```python
from build123d import *

# Parameters (mm, degrees)
SKETCH1_W                                    = 122
SKETCH1_H                                    = 43
BOSS_EXTRUDE1_DEPTH                          = 1.8
SKETCH2_W                                    = 9.05
SKETCH2_H                                    = 13.55
CUT_EXTRUDE1_DEPTH                           = 1.8
CSK_FOR_M3_COUNTERSUNK_FLAT_HEAD_SCR_2_COUNT = 2
CSK_FOR_M3_COUNTERSUNK_FLAT_HEAD_SCR_2_PITCH = 32.75
CSK_FOR_M3_COUNTERSUNK_FLAT_HEAD_SCR_3_COUNT = 2
CSK_FOR_M3_COUNTERSUNK_FLAT_HEAD_SCR_3_PITCH = 117.650169996
CSK_FOR_M3_COUNTERSUNK_FLAT_HEAD_SCR_4_COUNT = 2
CSK_FOR_M3_COUNTERSUNK_FLAT_HEAD_SCR_4_PITCH = 113
CUT_EXTRUDE2_DEPTH                           = 1.8
FILLET1_R                                    = 1
F_4_2_4_2_DIAMETER_HOLE1_D                   = 4.2
F_4_2_4_2_DIAMETER_HOLE1_DEPTH               = 1.8
F_4_2_4_2_DIAMETER_HOLE1_TIP                 = 1.2618073
CUT_EXTRUDE3_DEPTH                           = 1.8


with BuildPart() as part:
    # Sketch1 → Boss-Extrude1 (new body)
    with BuildSketch(Plane(origin=(0, 0, 0), x_dir=(0, 0, -1), z_dir=(1, 0, 0))):
        Rectangle(SKETCH1_W, SKETCH1_H)
    extrude(amount=BOSS_EXTRUDE1_DEPTH)

    # Sketch2 → Cut-Extrude1 (cut)
    with BuildSketch(Plane(origin=(1.8, 0, 0), x_dir=(0, 0, -1), z_dir=(1, 0, 0))):
        with Locations((-38.975, 0.005)):
            Rectangle(SKETCH2_W, SKETCH2_H)
    extrude(amount=-CUT_EXTRUDE1_DEPTH, mode=Mode.SUBTRACT)

    # Sketch3 → CSK for M3 Countersunk Flat Head Screw1 (revolve, cut)
    with BuildSketch(Plane(origin=(1.8, -15.5, 56.5), x_dir=(0, 0, -1), z_dir=(0, 1, 0))):
        Polygon((0, 0), (0, 1.8), (1.7, 1.8), (1.7, 1.7), (3.4, 0), align=None)
    csk_for_m3_countersunk_flat_head_screw1 = revolve(axis=Axis((8.15, -15.5, 56.5), (-1, 0, 0)), mode=Mode.SUBTRACT)

    # CSK for M3 Countersunk Flat Head Scr 2: CSK for M3 Countersunk Flat Head Screw1 ×2
    with Locations(*[(0, i * CSK_FOR_M3_COUNTERSUNK_FLAT_HEAD_SCR_2_PITCH, 0) for i in range(1, CSK_FOR_M3_COUNTERSUNK_FLAT_HEAD_SCR_2_COUNT)]):
        add(csk_for_m3_countersunk_flat_head_screw1, mode=Mode.SUBTRACT)

    # CSK for M3 Countersunk Flat Head Scr 3: CSK for M3 Countersunk Flat Head Screw1 ×2
    with Locations(*[Vector(0, 0.278367639, -0.9604746) * (i * CSK_FOR_M3_COUNTERSUNK_FLAT_HEAD_SCR_3_PITCH) for i in range(1, CSK_FOR_M3_COUNTERSUNK_FLAT_HEAD_SCR_3_COUNT)]):
        add(csk_for_m3_countersunk_flat_head_screw1, mode=Mode.SUBTRACT)

    # CSK for M3 Countersunk Flat Head Scr 4: CSK for M3 Countersunk Flat Head Screw1 ×2
    with Locations(*[(0, 0, -i * CSK_FOR_M3_COUNTERSUNK_FLAT_HEAD_SCR_4_PITCH) for i in range(1, CSK_FOR_M3_COUNTERSUNK_FLAT_HEAD_SCR_4_COUNT)]):
        add(csk_for_m3_countersunk_flat_head_screw1, mode=Mode.SUBTRACT)

    # Sketch5 → Cut-Extrude2 (cut)
    with BuildSketch(Plane(origin=(1.8, 0, 0), x_dir=(0, 0, -1), z_dir=(1, 0, 0))):
        Polygon((30.5, -12.9), (51, -12.9), (51, 3.9), (61, 3.9), (61, 7.9), (51, 7.9), (51, 13.9), (30.5, 13.9), align=None)
    extrude(amount=-CUT_EXTRUDE2_DEPTH, mode=Mode.SUBTRACT)

    # Fillet1
    fillet1_edges = [part.edges().sort_by_distance(p)[0] for p in [
        (0.9, 7.9, -61),
        (0.9, 3.9, -61),
        (0.9, 21.5, 61),
        (0.9, 21.5, -61),
        (0.9, -21.5, -61),
        (0.9, -21.5, 61),
    ]]
    fillet(fillet1_edges, radius=FILLET1_R)

    # Ø4.2 (4.2) Diameter Hole1
    with Locations(Plane(origin=(1.8, 0, 0), x_dir=(0, 0, -1), z_dir=(1, 0, 0))):
        with Locations((-14.5, 16), (17.5, 16), (17.5, -16), (-14.5, -16)):
            Hole(F_4_2_4_2_DIAMETER_HOLE1_D / 2, depth=F_4_2_4_2_DIAMETER_HOLE1_DEPTH)
            with Locations((0, 0, -(F_4_2_4_2_DIAMETER_HOLE1_DEPTH + F_4_2_4_2_DIAMETER_HOLE1_TIP / 2))):  # 118° drill point
                Cone(0, F_4_2_4_2_DIAMETER_HOLE1_D / 2, F_4_2_4_2_DIAMETER_HOLE1_TIP, mode=Mode.SUBTRACT)

    # Sketch8 → Cut-Extrude3 (cut)
    with BuildSketch(Plane(origin=(1.8, 0, 0), x_dir=(0, 0, -1), z_dir=(1, 0, 0))):
        with BuildLine():
            ThreePointArc((12.000022812, 15.984159355), (13.610912703, 12.110912703), (17.484159355, 10.500022812))
            ThreePointArc((17.484159355, 10.500022812), (18.064905248, 10.312049545), (18.428192241, 9.821516873))
            ThreePointArc((18.428192241, 9.821516873), (20.05, 0), (18.428192241, -9.821516873))
            ThreePointArc((18.428192241, -9.821516873), (18.064905248, -10.312049545), (17.484159355, -10.500022812))
            ThreePointArc((17.484159355, -10.500022812), (13.610912703, -12.110912703), (12.000022812, -15.984159355))
            ThreePointArc((12.000022812, -15.984159355), (11.812049545, -16.564905248), (11.321516873, -16.928192241))
            ThreePointArc((11.321516873, -16.928192241), (1.5, -18.55), (-8.321516873, -16.928192241))
            ThreePointArc((-8.321516873, -16.928192241), (-8.812049545, -16.564905248), (-9.000022812, -15.984159355))
            ThreePointArc((-9.000022812, -15.984159355), (-10.610912703, -12.110912703), (-14.484159355, -10.500022812))
            ThreePointArc((-14.484159355, -10.500022812), (-15.064905248, -10.312049545), (-15.428192241, -9.821516873))
            ThreePointArc((-15.428192241, -9.821516873), (-17.05, 0), (-15.428192241, 9.821516873))
            ThreePointArc((-15.428192241, 9.821516873), (-15.064905248, 10.312049545), (-14.484159355, 10.500022812))
            ThreePointArc((-14.484159355, 10.500022812), (-10.610912703, 12.110912703), (-9.000022812, 15.984159355))
            ThreePointArc((-9.000022812, 15.984159355), (-8.812049545, 16.564905248), (-8.321516873, 16.928192241))
            ThreePointArc((-8.321516873, 16.928192241), (1.5, 18.55), (11.321516873, 16.928192241))
            ThreePointArc((11.321516873, 16.928192241), (11.812049545, 16.564905248), (12.000022812, 15.984159355))
        make_face()
    extrude(amount=-CUT_EXTRUDE3_DEPTH, mode=Mode.SUBTRACT)


solid = part.part
```
Can you work these out from the model? Positions are in its coordinate system, mm. A direction names the side the tool comes from. Coordinates: 2 decimals unless noted, no trailing zeros. Loops run counter-clockwise (first coordinate to the right, second up) from the corner with the lowest first, then second, coordinate; pieces in that order, holes last.
1) For pin 1 (4.5 mm diameter, centred on y = 17.25, z = -56.5, fed in from +X); pin 2 (4 mm diameter, centred on y = -15.5, z = -56.5, fed in from +X), each with a flat end and sliding along its axis, tell me the tip position at first contact or that it passes through.
2) Imagine slicing it at D-D on y = 12.5. List the corners of the cut face in (x, z) for me, plus the area to 3 significant figures.
3) Imagine slicing it at B-B on z = -56.5. List the corners of the cut face in (x, y) for me.
4) Which directions (+Z, -Z, +X, -X, +Y, -Y) give clear straight access to the entire face, cutting with the end or side of a thin tool? Please do faces 4 (the cylindrical face through (0.91, 12.15, -13.57)), 5 (the conical face through (0.206, 17.942, -58.169)).
5) Thinking about a two-plate mould opening in Y: for faces 1 (the flat face through (1.8, -14, -13)), 2 (the cylindrical face through (0.89, 17.77, 15.63)), 3 (the conical face through (0.206, 17.942, 54.831)), which applies, pulls with the +Y half, pulls with the -Y half, needs draft (parallel to the pull), parting line crosses it, or undercut?
6) Imagine slicing it at A-A on z = -38. List the corners of the cut face in (x, y) for me.
7) Imagine slicing it at C-C on y = -4. List the corners of the cut face in (x, z) for me, plus the area to 3 significant figures.
8) I need wall thicknesses on probe 1 along Y at (x, z) = (1.1, -17.5); probe 2 along Y at (x, z) = (0.75, -0.5); probe 3 along Z at (x, y) = (0.6, 16.5). Which ranges of each line are inside material? Lowest first, please.
Completed:
1. pin 1: stops at x = 0.65
1. pin 2: stops at x = 0.4
2. outline: (0, -61) - (1.8, -61) - (1.8, -51) - (0, -51) - close; (0, -30.5) - (1.8, -30.5) - (1.8, -13.26) - (0, -13.26) - close; (0, 10.26) - (1.8, 10.26) - (1.8, 61) - (0, 61) - close
2. area: 140 mm2
3. outline: (0, -21.5) - (1.8, -21.5) - (1.8, -18.9) - (0.1, -17.2) - (0, -17.2) - close; (0, -13.8) - (0.1, -13.8) - (1.8, -12.1) - (1.8, 3.9) - (0, 3.9) - close; (0, 7.9) - (1.8, 7.9) - (1.8, 13.85) - (0.1, 15.55) - (0, 15.55) - close; (0, 18.95) - (0.1, 18.95) - (1.8, 20.65) - (1.8, 21.5) - (0, 21.5) - close
4. face 4: +X, -X
4. face 5: +X
5. face 1: needs draft
5. face 2: undercut
5. face 3: undercut
6. outline: (0, -21.5) - (1.8, -21.5) - (1.8, -12.9) - (0, -12.9) - close; (0, 13.9) - (1.8, 13.9) - (1.8, 21.5) - (0, 21.5) - close
7. outline: (0, -61) - (1.8, -61) - (1.8, -51) - (0, -51) - close; (0, -30.5) - (1.8, -30.5) - (1.8, -19.79) - (0, -19.79) - close; (0, 16.79) - (1.8, 16.79) - (1.8, 34.45) - (0, 34.45) - close; (0, 43.5) - (1.8, 43.5) - (1.8, 61) - (0, 61) - close
7. area: 101 mm2
8. probe 1: y = -21.5 to -18.1, -13.9 to -10.5, 10.5 to 13.9, 18.1 to 21.5
8. probe 2: y = -21.5 to -18.53, 18.53 to 21.5
8. probe 3: z = -61 to -58.57, -54.43 to -19.54, -15.46 to -11.85, 8.85 to 12.46, 16.54 to 54.43, 58.57 to 61
